Autodesk Inventor part; units mm, degrees
ref_plane "YZ Plane" through (0, 0, 0) normal (1, 0, 0) x (0, 1, 0)
ref_plane "XZ Plane" through (0, 0, 0) normal (0, 1, 0) x (-1, 0, 0)
ref_plane "Arbeitsebene1" through (0, 0, 1) normal (0, 0, 1) x (1, 0, 0)
sketch "Skizze1" plane through (0, 0, 1) normal (0, 0, 1) x (1, 0, 0)
  circle A0 centre (-16.4298, 19.2591) radius 1.4
  circle A1 centre (-3.4298, 6.2591) radius 1.4
  circle A2 centre (-3.4298, 32.2591) radius 1.4
  circle A3 centre (-3.43, 19.2591) radius 2.45 construction
  line L0 (-0.43, 35.2591) -> (-6.43, 35.2591)
  line L1 (-6.43, 35.2591) -> (-6.43, 3.2591)
  line L2 (-6.43, 3.2591) -> (-0.43, 3.2591)
  line L3 (-0.43, 3.2591) -> (-0.43, 35.2591)
  line L4 (-0.43, 35.2591) -> (-6.43, 3.2591) construction
  line L5 (-6.43, 35.2591) -> (-0.43, 3.2591) construction
  line L6 (-6.43, 22.7591) -> (-19.43, 22.7591)
  line L7 (-19.43, 22.7591) -> (-19.43, 15.7591)
  line L8 (-19.43, 15.7591) -> (-6.43, 15.7591)
  line L9 (-6.43, 15.7591) -> (-6.43, 22.7591)
  line L10 (-6.43, 22.7591) -> (-19.43, 15.7591) construction
  line L11 (-19.43, 22.7591) -> (-6.43, 15.7591) construction
  line L12 (-6.43, 3.2591) -> (-19.43, 15.7591)
  line L13 (-19.43, 22.7591) -> (-6.43, 35.2591)
  line L14 (-0.43, 3.2591) -> (3.27, 3.2591)
  line L15 (3.27, 3.2591) -> (3.27, 35.2591)
  line L16 (3.27, 35.2591) -> (-0.43, 35.2591)
  line L17 (-0.43, 35.2591) -> (-0.43, 3.2591)
  circle A4 centre (-3.43, 19.2591) radius 1.5
  point P0 (0, 0)
  point P1 (-12.93, 19.2591)
  point P2 (-6.43, 19.2591)
  dimension "d1" = 6
  dimension "d2" = 32
  dimension "d3" = 7
  dimension "d4" = 13
  dimension "d12" = 3.7
  dimension "d18" = 3
extrude "Extrusion1" add sketch "Skizze1" along normal blind 3.4
sketch "Skizze2" plane through (0, 0, 1) normal (0, 0, -1) x (-1, 0, 0)
  circle A0 centre (3.4298, 32.2591) radius 1.4
  line L0 (16.86, 34.56) -> (16.86, 4.56)
  circle A1 centre (16.4298, 19.2591) radius 1.4
  circle A2 centre (3.4298, 6.2591) radius 1.4
  line L1 (6.43, 35.2591) -> (19.43, 22.7591)
  line L2 (19.43, 22.7591) -> (19.43, 15.7591)
  line L3 (19.43, 15.7591) -> (6.43, 3.2591)
  circle A3 centre (16.4298, 19.2591) radius 1.4
  circle A4 centre (3.4298, 6.2591) radius 1.4
  circle A5 centre (3.4298, 32.2591) radius 1.4
  line L4 (-3.27, 29.2591) -> (12.67, 29.2591)
  line L5 (6.43, 35.2591) -> (19.43, 22.7591)
  line L6 (19.43, 22.7591) -> (19.43, 15.7591)
  line L7 (19.43, 22.7591) -> (13.43, 22.7591)
  line L8 (13.43, 22.7591) -> (13.43, 15.7591)
  line L9 (13.43, 15.7591) -> (19.43, 15.7591)
  line L10 (-3.27, 9.2591) -> (12.67, 9.2591)
  line L11 (19.43, 15.7591) -> (6.43, 3.2591)
  line L12 (6.43, 3.2591) -> (-3.27, 3.2591)
  line L13 (-3.27, 3.2591) -> (-3.27, 35.2591)
  line L14 (-3.27, 35.2591) -> (6.43, 35.2591)
  point P0 (0, 0)
  point P1 (12.67, 29.2591)
  dimension "d8" = 6
  dimension "d13" = 6
  dimension "d14" = 6
extrude "Extrusion2" add sketch "Skizze2" along normal blind 6.7 contours L7 L2 L9 L0 A1 | L0 A1 L9 L8 L7 | L4 L13 L14 L1 | L10 L3 L12 L13
sketch "Skizze4" plane through (0, 0, 1) normal (0, 0, -1) x (-1, 0, 0)
  circle A0 centre (3.43, 19.2591) radius 1.5
  circle A1 centre (3.43, 19.2591) radius 4
  point P0 (0, 0)
  dimension "d19" = 8
extrude "Extrusion4" cut sketch "Skizze4" against normal blind 3
properties part number "Assembly_Cube_Z_Focus_MGN_NEMA_belt_pushing_cage_v3"
Design review of the part built by this model. Coordinates are the model's own, in mm. A direction names the side the tool comes from. Coordinates: 2 decimals unless noted, no trailing zeros. Write each loop counter-clockwise with the first axis right and the second up, starting at its lowest first coordinate (ties: lowest second). Pieces come first, ordered by that corner, then holes.
1) Insertion check: pin 1 (2 mm diameter, centred on x = -10, z = -3.5, fed in from -Y); pin 2 (7 mm diameter, centred on x = -3.43, y = 19.26, fed in from -Z); pin 3 (5 mm diameter, centred on x = -17.5, z = -3, fed in from +Y). Each pin has a flat end and moves straight along its axis. Give the tip position at first contact, or say it passes through.
2) To check wall thickness, follow L1, parallel to Y at x = -5.25, z = -3.5; L2, parallel to Y at x = -4.25, z = 3; L3, parallel to X at y = 22, z = -4.5. State the ranges of each line that lie inside material, in increasing order.
3) Add section B-B (z = -0.25). Write out the cut boundary in (x, y), plus the area to 3 significant figures.
4) Add section D-D (z = 2.25). Write out the cut boundary in (x, y).
5) Add section A-A (x = -3.43). Write out the cut boundary in (y, z).
6) Machinability: for faces 1 (the cylindrical face through (-5.58, 22.63, 2.48)), 2 (the flat face through (-13.43, 19, -2)), 3 (the flat face through (-5, 29.259, -2)), which of the approach directions +Z, -Z, +X, -X, +Y, -Y give a long, thin tool a straight path to every point of the face, cutting with its end or side? Answer none if there is none.
7) Add section C-C (y = 31.5). Write out the cut boundary in (x, z).
8) Mouldability with a two-part tool opening along Y and no side actions: class faces 4 (the flat face through (-18, 20, -5.7)), 5 (the flat face through (-5.2, 19.3, 4)), 6 (the flat face through (-11.39, 8.03, 0.4)) as +Y half, -Y half, draft (parallel to the pull), parting line (faces both ways), or undercut.
Check result:
1. pin 1: stops at y = 5.73
1. pin 2: stops at z = 4
1. pin 3: stops at y = 22.76
2. L1: y = 3.26 to 9.26, 29.26 to 35.26
2. L2: y = 3.26 to 5.12, 7.39 to 15.34, 23.17 to 31.12, 33.39 to 35.26
2. L3: x = -19.43 to -13.43
3. outline: (-19.43, 15.76) - (-13.43, 15.76) - (-13.43, 22.76) - (-19.43, 22.76) - close; (-12.67, 9.26) - (-6.43, 3.26) - (3.27, 3.26) - (3.27, 9.26) - close; (-12.67, 29.26) - (3.27, 29.26) - (3.27, 35.26) - (-6.43, 35.26) - close; hole circle Ø2.8 at (-16.43, 19.26); hole circle Ø2.8 at (-3.43, 6.26); hole circle Ø2.8 at (-3.43, 32.26)
3. area: 177 mm2
4. outline: (-19.43, 15.76) - (-6.43, 3.26) - (3.27, 3.26) - (3.27, 35.26) - (-6.43, 35.26) - (-19.43, 22.76) - close; hole circle Ø2.8 at (-16.43, 19.26); hole circle Ø8 at (-3.43, 19.26); hole circle Ø2.8 at (-3.43, 6.26); hole circle Ø2.8 at (-3.43, 32.26)
5. outline: (3.26, -5.7) - (4.86, -5.7) - (4.86, 4.4) - (3.26, 4.4) - close; (7.66, -5.7) - (9.26, -5.7) - (9.26, 1) - (15.26, 1) - (15.26, 4) - (17.76, 4) - (17.76, 4.4) - (7.66, 4.4) - close; (20.76, 4) - (23.26, 4) - (23.26, 1) - (29.26, 1) - (29.26, -5.7) - (30.86, -5.7) - (30.86, 4.4) - (20.76, 4.4) - close; (33.66, -5.7) - (35.26, -5.7) - (35.26, 4.4) - (33.66, 4.4) - close
6. face 1: -Z
6. face 2: -Z, +X, +Y, -Y
6. face 3: -Z, +X, -X
7. outline: (-10.34, -5.7) - (-4.61, -5.7) - (-4.61, 4.4) - (-10.34, 4.4) - close; (-2.25, -5.7) - (3.27, -5.7) - (3.27, 4.4) - (-2.25, 4.4) - close
8. face 4: draft
8. face 5: undercut
8. face 6: -Y half
